For this review, take the finished solid that the model builds, in its own axes (mm). Coordinates: 2 decimals unless noted, no trailing zeros. Loops run counter-clockwise (first coordinate to the right, second up) from the corner with the lowest first, then second, coordinate; pieces in that order, holes last. Notation, with made-up numbers: M 41.5,60 L 100.5,60 A27 cw 100.5,84 Z; hole C -0.75,45.25 d8. An arc over 180 degrees is marked long. Answer as a JSON object with one key per item and string values. Group by question number.
Item 1: Insertion check: pin 1 (11.5 mm diameter, centred on x = -377, z = 962, fed in from -Y). The pin has a flat end and moves straight along its axis. Give the tip position at first contact, or say it passes through.
Item 2: Wall thickness on L1, parallel to X at y = 13, z = -962; L2, parallel to X at y = 13.5, z = 606; L3, parallel to Z at x = -116, y = 23.25: over which ranges is each line inside the solid? List them lowest first. Write a range as from..to.
Item 3: Add section B-B (z = -352). State the section outline as (x, y) points, then the cut area to 3 significant figures.
Item 4: Add section A-A (x = 310.5). State the section outline as (y, z) points.
Item 5: Add section C-C (z = 504). State the section outline as (x, y) points (3 decimals).
from build123d import *

# Parameters (mm, degrees)
CROQUIS1_W                 = 600
CROQUIS1_H                 = 1500
CROQUIS1_W_2               = 560
CROQUIS1_H_2               = 1460
SALIENTE_EXTRUIR1_DEPTH    = 20
CROQUIS2_R                 = 5
CORTAR_EXTRUIR1_DEPTH      = 15
REDONDEO1_R                = 2
CORTAR_EXTRUIR2_DEPTH      = 575
CORTAR_EXTRUIR2_DEPTH_BACK = 15
CROQUIS5_R                 = 5
CROQUIS5_R_2               = 3.75
SALIENTE_EXTRUIR2_DEPTH    = 15
ESCALA1_SCALE              = 1.3


with BuildPart() as part:
    # Croquis1 → Saliente-Extruir1 (new body)
    with BuildSketch(Plane(origin=(0, 0, 0), x_dir=(1, 0, 0), z_dir=(0, 1, 0))):
        Rectangle(CROQUIS1_W, CROQUIS1_H)
        Rectangle(CROQUIS1_W_2, CROQUIS1_H_2, mode=Mode.SUBTRACT)
    extrude(amount=SALIENTE_EXTRUIR1_DEPTH)

    # Croquis2 → Cortar-Extruir1 (cut)
    with BuildSketch(Plane.XZ):
        with Locations((-290, 740)):
            Circle(CROQUIS2_R)
        with Locations((290, 740)):
            Circle(CROQUIS2_R)
        with Locations((290, -740)):
            Circle(CROQUIS2_R)
        with Locations((-290, -740)):
            Circle(CROQUIS2_R)
    extrude(amount=-CORTAR_EXTRUIR1_DEPTH, mode=Mode.SUBTRACT)

    # Redondeo1
    redondeo1_edges = [part.edges().sort_by_distance(p)[0] for p in [
        (-300, 20, 0),
        (280, 20, 0),
        (0, 20, 750),
        (0, 20, -730),
        (-280, 20, 0),
        (0, 20, 730),
        (300, 20, 0),
        (0, 20, -750),
    ]]
    fillet(redondeo1_edges, radius=REDONDEO1_R)

    # Croquis4 → Cortar-Extruir2 (cut, two sides)
    with BuildSketch(Plane.ZY.offset(-280)) as cortar_extruir2_sk:
        with BuildLine():
            Line((600, 12.75), (100, 12.75))
            Line((100, 12.75), (100, 5.25))
            Line((100, 5.25), (600, 5.25))
            ThreePointArc((600, 5.25), (603.75, 9), (600, 12.75))
        make_face()
        with BuildLine():
            Line((100, 5.25), (100, 12.75))
            ThreePointArc((100, 12.75), (96.25, 9), (100, 5.25))
        make_face()
    extrude(amount=CORTAR_EXTRUIR2_DEPTH, mode=Mode.SUBTRACT)
    extrude(cortar_extruir2_sk.sketch, amount=-CORTAR_EXTRUIR2_DEPTH_BACK, mode=Mode.SUBTRACT)

    # Croquis5 → Saliente-Extruir2 (add)
    with BuildSketch(Plane.ZY.offset(-280)):
        with Locations((-596.25, 9)):
            Circle(CROQUIS5_R)
        with Locations((-596.25, 9)):
            Circle(CROQUIS5_R_2, mode=Mode.SUBTRACT)
    saliente_extruir2 = extrude(amount=SALIENTE_EXTRUIR2_DEPTH)

    # Simetría1: Saliente-Extruir2 across plane
    add(saliente_extruir2.mirror(Plane(origin=(0, 0, 0), x_dir=(0, 0, 1), z_dir=(1, 0, 0))))


with BuildPart() as part_1:
    # Escala1: scaled about (0, 0, 0)
    add(part.part.scale(ESCALA1_SCALE))


solid = part_1.part
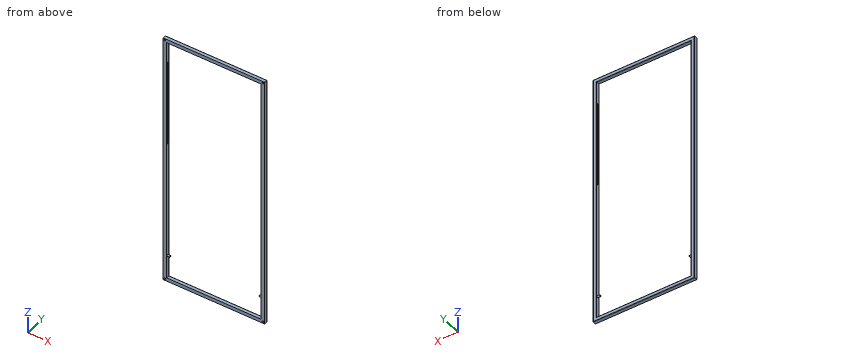
From the geometry:
{
 "1": {"pin 1": "stops at y = 19.5"},
 "2": {"L1": "x = -390..-383.5, -370.5..370.5, 383.5..390", "L2": "x = -390..-383.5, 383.5..390", "L3": "z = -975..-949, 949..975"},
 "3": {"outline": "M -390,0 L -364,0 L -364,23.4 A2.6 ccw -366.6,26 L -387.4,26 A2.6 ccw -390,23.4 Z; M 364,0 L 390,0 L 390,23.4 A2.6 ccw 387.4,26 L 366.6,26 A2.6 ccw 364,23.4 Z", "area": "1,350 mm²"},
 "4": {"outline": "M 0,-975 L 23.4,-975 A2.6 ccw 26,-972.4 L 26,-951.6 A2.6 ccw 23.4,-949 L 0,-949 Z; M 0,949 L 23.4,949 A2.6 ccw 26,951.6 L 26,972.4 A2.6 ccw 23.4,975 L 0,975 Z"},
 "5": {"outline": "M -390,0 L -364,0 L -364,6.825 L -383.5,6.825 L -383.5,16.575 L -364,16.575 L -364,23.4 A2.6 ccw -366.6,26 L -387.4,26 A2.6 ccw -390,23.4 Z; M 364,0 L 390,0 L 390,23.4 A2.6 ccw 387.4,26 L 366.6,26 A2.6 ccw 364,23.4 L 364,16.575 L 383.5,16.575 L 383.5,6.825 L 364,6.825 Z"}
}
